Build history of the part. All positions in model axes, mm. Give positions to 0.01 mm unless a question says otherwise; leave off trailing zeros. Loops run counter-clockwise (first coordinate to the right, second up) from the corner with the lowest first, then second, coordinate; pieces in that order, holes last. Notation, with made-up numbers: (14, -17.5) -> (49, -17.5) arc R17 cw to (49, 6.5) -> close; hole circle Ø1 at (33.25, 42.5). An arc over 180 degrees is marked (long way). Answer as a JSON object with one key per item and string values. Group by question number.
from build123d import *

# Parameters (mm, degrees)
SKETCH1_W                = 38.1
SKETCH1_H                = 38.1
BOSS_EXTRUDE1_DEPTH      = 21.336
SKETCH2_W                = 35.814
SKETCH2_H                = 19.05
CUT_EXTRUDE1_DEPTH       = 48.641761051
HOLE1_D                  = 12.7254
HOLE1_DEPTH              = 21.336
M3_CLEARANCE_HOLE1_D     = 3.556
M3_CLEARANCE_HOLE1_DEPTH = 21.336
M3_CLEARANCE_HOLE2_D     = 3.556
M3_CLEARANCE_HOLE2_DEPTH = 38.1


with BuildPart() as part:
    # Sketch1 → Boss-Extrude1 (new body)
    with BuildSketch(Plane(origin=(0, 21.336, 0), x_dir=(1, 0, 0), z_dir=(0, 1, 0))):
        Rectangle(SKETCH1_W, SKETCH1_H)
    extrude(amount=-BOSS_EXTRUDE1_DEPTH)

    # Sketch2 → Cut-Extrude1 (cut, through all)
    with BuildSketch(Plane.ZY.offset(19.05)):
        with Locations((-1.143, 11.811)):
            Rectangle(SKETCH2_W, SKETCH2_H)
    extrude(amount=-CUT_EXTRUDE1_DEPTH, mode=Mode.SUBTRACT)

    # Hole1
    with Locations(Plane(origin=(0, 0, 0), x_dir=(-1, 0, 0), z_dir=(0, -1, 0))):
        with Locations((0, 0)):
            Hole(HOLE1_D / 2, depth=HOLE1_DEPTH)

    # M3 Clearance Hole1
    with Locations(Plane(origin=(0, 0, 0), x_dir=(-1, 0, 0), z_dir=(0, -1, 0))):
        with Locations((6.914797213, -12.135202787), (13.470384182, 13.470384182), (-13.470384182, 13.470384182), (0, -9.779), (6.914797213, -6.914797213), (9.779, 0), (6.914797213, 6.914797213), (0, 9.779), (-6.914797213, 6.914797213), (-9.779, 0), (-6.914797213, -6.914797213), (-13.470384182, -5.579615818), (-6.914797213, -12.135202787), (-13.470384182, -13.470384182), (-13.470384182, 5.579615818), (-6.914797213, 12.135202787), (13.470384182, 5.579615818), (6.914797213, 12.135202787), (13.470384182, -5.579615818), (13.470384182, -13.470384182)):
            Hole(M3_CLEARANCE_HOLE1_D / 2, depth=M3_CLEARANCE_HOLE1_DEPTH)

    # M3 Clearance Hole2
    with Locations(Plane.XY.offset(19.05)):
        with Locations((-6.92785, 14.42212), (13.470382, 7.86638), (13.470382, 15.75562), (6.92785, 9.19988), (6.92785, 14.42212), (0, 11.811), (-13.470382, 7.86638), (-13.470382, 15.75562), (-6.92785, 9.19988)):
            Hole(M3_CLEARANCE_HOLE2_D / 2, depth=M3_CLEARANCE_HOLE2_DEPTH)


solid = part.part
(1) Pin check, flat tips, straight feed: pin 1 (5.5 mm diameter, centred on x = -9.779, z = 0, fed in from +Y); pin 2 (4 mm diameter, centred on x = 13.47, y = 7.87, fed in from -Z). Stop position of each tip, or through.
(2) Probe line 1 along Z through (x, y) = (-5.5, 2.5); line 2 along Y through (x, z) = (-6, -8.5); line 3 along X through (y, z) = (8.75, 17). List the from-to ranges inside material, lowest first. Write a range as [from, to].
(3) Saw through at D-D on y = 3. List the corners of the cut face in (x, z).
(4) Saw through at C-C on x = 13.5. Give the number of separate pieces and of enclosed holes in the cut face, plus the area to 3 significant figures.
(5) Saw through at A-A on x = 0. List the corners of the cut face in (y, z).
(6) Saw through at B-B on z = 0. List the corners of the cut face in (x, y).
(7) Pull direction Z, two halves, no side cores. Call faces 1 (the cylindrical face through (5.604, 1.159, 10.934)), 2 (the flat face through (0, 8, 19.05)), 3 (the flat face through (-5, 0, -5)): pulls with the +Z half, pulls with the -Z half, needs draft (parallel to the pull), parting line crosses it, or undercut.
Calculated:
{
 "1": {"pin 1": "stops at y = 2.29", "pin 2": "stops at z = 16.76"},
 "2": {"line 1": "z = [16.76, 19.05]", "line 2": "y = [0, 2.29]", "line 3": "x = [-19.05, -15.01], [-11.93, -8.65], [-5.21, 5.21], [8.65, 11.93], [15.01, 19.05]"},
 "3": {"outline": "(-19.05, 16.76) -> (19.05, 16.76) -> (19.05, 19.05) -> (-19.05, 19.05) -> close"},
 "4": {"separate pieces": "7", "enclosed holes": "0", "area": "81.9 mm^2"},
 "5": {"outline": "(0, -19.05) -> (2.29, -19.05) -> (2.29, -11.56) -> (0, -11.56) -> close; (0, -8) -> (2.29, -8) -> (2.29, -6.36) -> (0, -6.36) -> close; (0, 6.36) -> (2.29, 6.36) -> (2.29, 8) -> (0, 8) -> close; (0, 11.56) -> (2.29, 11.56) -> (2.29, 16.76) -> (10.03, 16.76) -> (10.03, 19.05) -> (0, 19.05) -> close; (13.59, 16.76) -> (21.34, 16.76) -> (21.34, 19.05) -> (13.59, 19.05) -> close"},
 "6": {"outline": "(-19.05, 0) -> (-11.56, 0) -> (-11.56, 2.29) -> (-19.05, 2.29) -> close; (-8, 0) -> (-6.36, 0) -> (-6.36, 2.29) -> (-8, 2.29) -> close; (6.36, 0) -> (8, 0) -> (8, 2.29) -> (6.36, 2.29) -> close; (11.56, 0) -> (19.05, 0) -> (19.05, 2.29) -> (11.56, 2.29) -> close"},
 "7": {"face 1": "undercut", "face 2": "pulls with the +Z half", "face 3": "needs draft"}
}
